Read the model definition and answer for the solid it produces. Units are mm, in the model's axes. Face numbers are marked on the shaded views. Round coordinates to 2 decimals unless told otherwise and drop trailing zeros. Order: outer loops, then holes, each group sorted by start corner. A loop starts at its lowest first (then second) coordinate and runs counter-clockwise, first axis right, second up. Notation, with made-up numbers: M 9,44.25 L 42,44.25 A31 ccw 42,74.25 Z; hole C 0.25,83.5 d1. An arc over 180 degrees is marked long. Answer as CSV lines item,"result".
```python
from build123d import *

# Parameters (mm, degrees)
F0_W     = 450
F0_H     = 450
F1_DEPTH = 950
F2_W     = 50
F2_H     = 50
F2_H_2   = 425
F2_W_2   = 330
F3_DEPTH = 450.001
F4_W     = 380
F4_H     = 425
F5_DEPTH = 450.001
F6_W     = 380
F6_H     = 75
F6_H_2   = 275
F7_DEPTH = 135.7561676147


with BuildPart() as f1:
    # F0 (on Top) → F1 (new body)
    with BuildSketch(Plane.XY):
        Rectangle(F0_W, F0_H)
    extrude(amount=F1_DEPTH)

    # F2 (on face) → F3 (cut, through all)
    with BuildSketch(Plane.YZ.offset(225)):
        Polygon((-225, 950), (-225, 475), (140, 475), (191.5523596896, 950), align=None)
        Polygon((225, 935.6966614723), (175, 475), (225, 475), align=None)
        with Locations((200, 450)):
            Rectangle(F2_W, F2_H)
        with Locations((200, 212.5)):
            Rectangle(F2_W, F2_H_2)
        with Locations((-25, 212.5)):
            Rectangle(F2_W_2, F2_H_2)
    extrude(amount=-F3_DEPTH, mode=Mode.SUBTRACT)

    # F4 (on face) → F5 (cut, through all)
    with BuildSketch(Plane.XZ.offset(225)):
        with Locations((0, 212.5)):
            Rectangle(F4_W, F4_H)
    extrude(amount=-F5_DEPTH, mode=Mode.SUBTRACT)

    # F6 (on face) → F7 (cut, through all)
    with BuildSketch(Plane(origin=(0, 87.4179409303, -9.4875813351), x_dir=(1, 0, 0), z_dir=(0, -0.9941620044, 0.1078976784))):
        with Locations((0, 849.8326270669)):
            Rectangle(F6_W, F6_H)
        with Locations((0, 624.8326270669)):
            Rectangle(F6_W, F6_H_2)
    extrude(amount=-F7_DEPTH, mode=Mode.SUBTRACT)


solid = f1.part
```
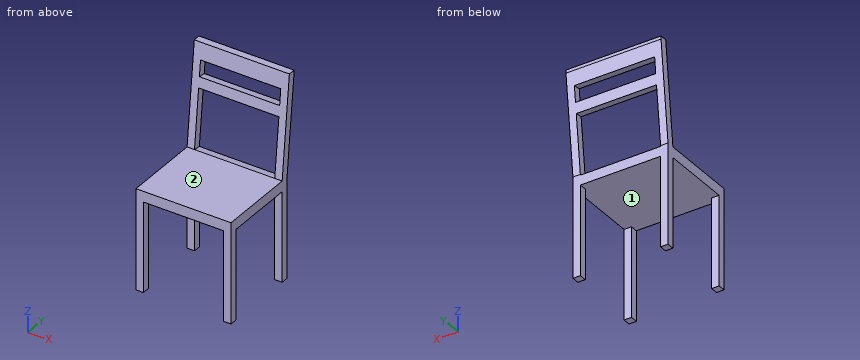
Item 1: Determine the mould class of the marked faces 1 and 2 for opening direction X: +X half, -X half, draft (parallel to the pull), parting line (faces both ways), or undercut.
Ans:
face 1,"undercut"
face 2,"draft"
Item 2: A cutting plane is placed at A-A, the plane z = 264. Determine the outline of the cut face in (x, y).
Ans:
outline,"M -225,-225 L -190,-225 L -190,-190 L -225,-190 Z; M -225,140 L -190,140 L -190,175 L -225,175 Z; M 190,-225 L 225,-225 L 225,-190 L 190,-190 Z; M 190,140 L 225,140 L 225,175 L 190,175 Z"
Item 3: Find the intervals of material crossed by probe 1 along X at (y, z) = (167, 533); probe 2 along Z at (x, y) = (68.5, 6); probe 3 along Y at (x, z) = (-195, 463.5), in increasing order. Write a range as [from, to].
Ans:
probe 1,"[-225, -190], [190, 225]"
probe 2,"[425, 475]"
probe 3,"[-225, 175]"
Item 4: A cutting plane is placed at D-D, the plane y = 155. Determine the outline of the cut face in (x, z).
Ans:
outline,"M -225,0 L -190,0 L -190,425 L 190,425 L 190,0 L 225,0 L 225,613.21 L 190,613.21 L 190,473.37 L -190,473.37 L -190,613.21 L -225,613.21 Z"
Item 5: Flat-ended cylindrical pins translate along their axes: pin 1 (2 mm diameter, centred on x = -127, y = 101, fed in from -Z); pin 2 (1 mm diameter, centred on x = 72.5, y = 97, fed in from +Z). Find the tip coordinate at first contact, or state that the pin passes through.
Ans:
pin 1,"z = 425"
pin 2,"z = 475"
Item 6: A cutting plane is placed at B-B, the plane x = -131.5. Determine the outline of the cut face in (y, z), and give its area (3 significant figures).
Ans:
outline,"M -225,425 L 175,425 L 175,471.2 L 140,475 L -225,475 Z; M 169.67,748.39 L 204.26,744.64 L 209.66,794.35 L 175.07,798.1 Z; M 183.16,872.66 L 217.75,868.91 L 225,935.7 L 225,950 L 191.55,950 Z"
area,"24,400 mm2"
Item 7: A cutting plane is placed at C-C, the plane z = 605. Determine the outline of the cut face in (x, y).
Ans:
outline,"M -225,154.11 L -190,154.11 L -190,189.11 L -225,189.11 Z; M 190,154.11 L 225,154.11 L 225,189.11 L 190,189.11 Z"
